```python
from build123d import *

# Parameters (mm, degrees)
F1_R   = 8
F1_R_2 = 6


with BuildPart() as f2:
    # F2: sweep along a path in F0
    with BuildLine(Plane.XZ) as f2_path:
        Line((-15.5, 0), (-15.5, 25))
        ThreePointArc((-15.5, 25), (-10.960155, 35.960155), (0, 40.5))
        ThreePointArc((0, 40.5), (10.960155, 35.960155), (15.5, 25))
        Line((15.5, 25), (15.5, 0))
    # F1 (on Top) → F2 (sweep)
    with BuildSketch(Plane.XY):
        with Locations((-15.5, 0)):
            Circle(F1_R)
        with Locations((-15.5, 0)):
            Circle(F1_R_2, mode=Mode.SUBTRACT)
    sweep(path=f2_path.line)


solid = f2.part
```
CAD build for the part. Positions are in the model's coordinates, mm. A direction names the side the tool comes from. Give positions to 0.01 mm unless a question says otherwise; leave off trailing zeros. Put each result on its own line as item: value. Start each with the question number.
(1) Which spindle directions (+Z, -Z, +X, -X, +Y, -Y) get a long thin tool onto all of the face, cutting with end or side? Do faces 3 (the flat face through (14, 6, 0)), 4 (the cylindrical face through (-21.849, -4.868, 12.675)). Say none if no direction does.
(2) Flat gauge pins, fed straight in: pin 1 Ø4 at (y, z) = (-1.5, 38.5) entering from -X; pin 2 Ø1.5 at (y, z) = (-3, 32.5) entering from -X; pin 3 Ø10 at (x, z) = (11.5, 27) entering from -Y; pin 4 Ø10 at (x, z) = (-7.5, 8) entering from +Y. Where does each tip first touch, or does it go through?
(3) Saw through at A-A, the plane z = 7. Give the number of separate pieces and of enclosed holes in the cut face, then the cut area to 3 significant figures.
(4) Mould opens along X. For faces 1 (the cylindrical face through (-9.96, -2.3, 12.68)), 2 (the flat face through (-14, 6, 0)) say: +X half, -X half, draft (parallel to the pull), parting line (faces both ways), or undercut.
(5) Drill centre lines: line 1 along X through (y, z) = (-5.5, 13); line 2 along X through (y, z) = (-2.25, 21); line 3 along Z through (x, y) = (-2, 0.5). Where is each one in solid material? Low to high.
Check result:
1. face 3: -Z, +X, -X, +Y, -Y
1. face 4: -Z
2. pin 1: stops at x = -20.39
2. pin 2: stops at x = -22.03
2. pin 3: stops at y = -8
2. pin 4: stops at y = 7.42
3. separate pieces: 2
3. enclosed holes: 2
3. area: 176 mm2
4. face 1: undercut
4. face 2: draft
5. line 1: x = -21.31 to -17.9, -13.1 to -9.69, 9.69 to 13.1, 17.9 to 21.31
5. line 2: x = -23.18 to -21.06, -9.94 to -7.82, 7.82 to 9.94, 21.06 to 23.18
5. line 3: z = 32.24 to 34.31, 46.39 to 48.4
